from build123d import *

# Parameters (mm, degrees)
F0_R     = 9.525
F0_R_2   = 63.5
F0_R_3   = 31.75
F0_R_4   = 19.05
F0_R_5   = 6.35
F1_DEPTH = 19.05
F2_DEPTH = 76.2
F3_DEPTH = 50.8
F4_DEPTH = 38.1


with BuildPart() as f1:
    # F0 (on Top) → F1 (new body)
    with BuildSketch(Plane.XY):
        with BuildLine():
            ThreePointArc((0, 76.2), (53.881537, 53.881537), (76.2, 0))
            ThreePointArc((76.2, 0), (53.881537, -53.881537), (0, -76.2))
            Line((0, -76.2), (88.9, -76.2))
            Line((88.9, -76.2), (107.95, -76.2))
            ThreePointArc((107.95, -76.2), (127, -57.15), (107.95, -38.1))
            Line((107.95, -38.1), (88.9, -38.1))
            Line((88.9, -38.1), (88.9, 38.1))
            Line((88.9, 38.1), (107.95, 38.1))
            ThreePointArc((107.95, 38.1), (127, 57.15), (107.95, 76.2))
            Line((107.95, 76.2), (88.9, 76.2))
            Line((88.9, 76.2), (0, 76.2))
        make_face()
        with Locations((107.95, -57.15)):
            Circle(F0_R, mode=Mode.SUBTRACT)
        with Locations((107.95, 57.15)):
            Circle(F0_R, mode=Mode.SUBTRACT)
        with BuildLine():
            ThreePointArc((0, -76.2), (-76.2, 0), (0, 76.2))
            Line((0, 76.2), (-88.9, 76.2))
            Line((-88.9, 76.2), (-107.95, 76.2))
            ThreePointArc((-107.95, 76.2), (-127, 57.15), (-107.95, 38.1))
            Line((-107.95, 38.1), (-88.9, 38.1))
            Line((-88.9, 38.1), (-88.9, -38.1))
            Line((-88.9, -38.1), (-107.95, -38.1))
            ThreePointArc((-107.95, -38.1), (-127, -57.15), (-107.95, -76.2))
            Line((-107.95, -76.2), (-88.9, -76.2))
            Line((-88.9, -76.2), (0, -76.2))
        make_face()
        with Locations((-107.95, -57.15)):
            Circle(F0_R, mode=Mode.SUBTRACT)
        with Locations((-107.95, 57.15)):
            Circle(F0_R, mode=Mode.SUBTRACT)
        Circle(F0_R_2)
        Circle(F0_R_3, mode=Mode.SUBTRACT)
        Circle(F0_R_3)
        Circle(F0_R_4, mode=Mode.SUBTRACT)
        Circle(F0_R_4)
        Circle(F0_R_5, mode=Mode.SUBTRACT)
        Circle(F0_R_5)
    extrude(amount=F1_DEPTH)

    # F0 (on Top) → F2 (join)
    with BuildSketch(Plane.XY):
        with BuildLine():
            ThreePointArc((0, -76.2), (53.881537, -53.881537), (76.2, 0))
            ThreePointArc((76.2, 0), (53.881537, 53.881537), (0, 76.2))
            ThreePointArc((0, 76.2), (-76.2, 0), (0, -76.2))
        make_face()
        Circle(F0_R_2, mode=Mode.SUBTRACT)
    extrude(amount=F2_DEPTH)

    # F0 (on Top) → F3 (join)
    with BuildSketch(Plane.XY):
        Circle(F0_R_3)
        Circle(F0_R_4, mode=Mode.SUBTRACT)
    extrude(amount=F3_DEPTH)

    # F0 (on Top) → F4 (join)
    with BuildSketch(Plane.XY):
        Circle(F0_R_4)
        Circle(F0_R_5, mode=Mode.SUBTRACT)
    extrude(amount=F4_DEPTH)


solid = f1.part
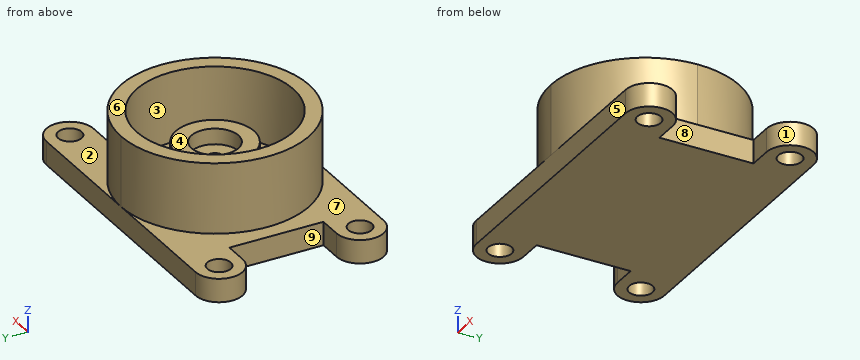
Here's how the part is built. I have some questions about the finished solid (model axes, mm). Face numbers are marked on the shaded views. A direction names the side the tool comes from. Coordinates: 2 decimals unless noted, no trailing zeros. Order: outer loops, then holes, each group sorted by start corner. A loop starts at its lowest first (then second) coordinate and runs counter-clockwise, first axis right, second up. Notation, with made-up numbers: M -22,76.25 L 15,76.25 A9 ccw 15,92.25 Z; hole C 41.5,43 d7. An arc over 180 degrees is marked long. Answer as CSV lines item,"result". Start each with the question number.
1. I want a section at C-C, the plane x = -59. Write out the boundary of the cut face in (y, z), and give its area (3 significant figures).
2. I need wall thicknesses on line 1 (Y direction, x = 107, z = 6); line 2 (Y direction, x = 107.95, z = 6) (3 decimals); line 3 (X direction, y = -65.5, z = 7). Which ranges of each line are inside material? Lowest first, please. Write a range as [from, to].
3. For pin 1 (6 mm diameter, centred on x = 78.5, y = 43, fed in from +Z); pin 2 (21 mm diameter, centred on y = 11, z = 6.5, fed in from -X); pin 3 (10 mm diameter, centred on y = 13, z = 36, fed in from +X), each with a flat end and sliding along its axis, tell me the tip position at first contact or that it passes through.
4. On a 3-axis mill with a long thin cutter (end or side, diameter ignored), from which of +Z, -Z, +X, -X, +Y, -Y can I reach the whole of each face in a straight line? I mean the marked faces 5, 6, 7, 8 and 9. Say none if no direction works.
5. I want a section at A-A, the plane z = 26.5. Write out the boundary of the cut face in (x, y), and give its area (3 significant figures).
6. I want a section at B-B, the plane y = 57.15. Write out the boundary of the cut face in (x, z) (3 decimals), and give its area (3 significant figures).
7. We'd pull the mould along X, two halves only. Please class the marked faces 1, 2, 3 and 4: released by +X, released by -X, zero draft, split by the parting line, or undercut.
Recorded:
1,outline,"M -76.2,0 L 76.2,0 L 76.2,19.05 L 48.22,19.05 L 48.22,76.2 L 23.48,76.2 L 23.48,19.05 L -23.48,19.05 L -23.48,76.2 L -48.22,76.2 L -48.22,19.05 L -76.2,19.05 Z"
1,area,"5,730 mm2"
2,line 1,"y = [-76.2, -66.63], [-47.67, -38.1], [38.1, 47.67], [66.63, 76.2]"
2,line 2,"y = [-76.2, -66.675], [-47.625, -38.1], [38.1, 47.625], [66.675, 76.2]"
2,line 3,"x = [-125.07, -112.53], [-103.37, 103.37], [112.53, 125.07]"
3,pin 1,"stops at z = 19.05"
3,pin 2,"stops at x = -88.9"
3,pin 3,"stops at x = 75.78"
4,face 5,"+Z, -Z, +X, -X, -Y"
4,face 6,"+Z, +X, -X, +Y, -Y"
4,face 7,"+Z, -X"
4,face 8,"+Z, -Z, +X"
4,face 9,"+Z, -Z, -X"
5,outline,"C 0,0 d63.5; M 0,-76.2 A76.2 ccw 76.2,0 A76.2 ccw long Z; hole C 0,0 d127; hole C 0,0 d12.7"
5,area,"8,610 mm2"
6,outline,"M -127,0 L -117.475,0 L -117.475,19.05 L -127,19.05 Z; M -98.425,0 L 98.425,0 L 98.425,19.05 L 50.402,19.05 L 50.402,76.2 L 27.679,76.2 L 27.679,19.05 L -27.679,19.05 L -27.679,76.2 L -50.402,76.2 L -50.402,19.05 L -98.425,19.05 Z; M 117.475,0 L 127,0 L 127,19.05 L 117.475,19.05 Z"
6,area,"6,710 mm2"
7,face 1,"released by +X"
7,face 2,"zero draft"
7,face 3,"undercut"
7,face 4,"undercut"
